Autodesk Inventor part; units mm, degrees
ref_plane "YZ Plane" through (0, 0, 0) normal (1, 0, 0) x (0, 1, 0)
ref_plane "XZ Plane" through (0, 0, 0) normal (0, 1, 0) x (-1, 0, 0)
ref_plane "XY Plane" through (0, 0, 0) normal (0, 0, 1) x (1, 0, 0)
sketch "Sketch1" plane through (0, 0, 0) normal (0, 1, 0) x (-1, 0, 0)
  line L0 (0.25, 0.25) -> (-0.25, 0.25)
  line L1 (-0.25, 0.25) -> (-0.25, -0.25)
  line L2 (-0.25, -0.25) -> (0.25, -0.25)
  line L3 (0.25, -0.25) -> (0.25, 0.25)
  line L4 (0.25, 0.25) -> (-0.25, -0.25) construction
  line L5 (-0.25, 0.25) -> (0.25, -0.25) construction
  point P0 (0, 0)
  dimension "d0" = 0.5
  dimension "d1" = 0.5
extrude "Extrusion1" add sketch "Sketch1" along normal blind 11.75
sketch "Sketch2" plane through (-0.25, 0, 0.25) normal (0, 0, 1) x (1, 0, 0)
  line L0 (0, 0) -> (0.5, 0)
  line L1 (0.5, 0) -> (0.5, 11.75)
  line L2 (0, 11.75) -> (0.5, 11.75)
  line L3 (0, 0) -> (0, 11.75)
  line L4 (0, 11.75) -> (0.5, 11.75)
  line L5 (0.5, 11.75) -> (0.5, 11.25)
  line L6 (0.5, 11.25) -> (0, 11.25)
  line L7 (0, 11.25) -> (0, 11.75)
  point P0 (0.25, 0)
  point P1 (0, 11.25)
  dimension "d10" = 0.5
extrude "Extrusion2" add sketch "Sketch2" along normal blind 3.3 contours L3 L2 L1 L6
properties part number "switch-wire"
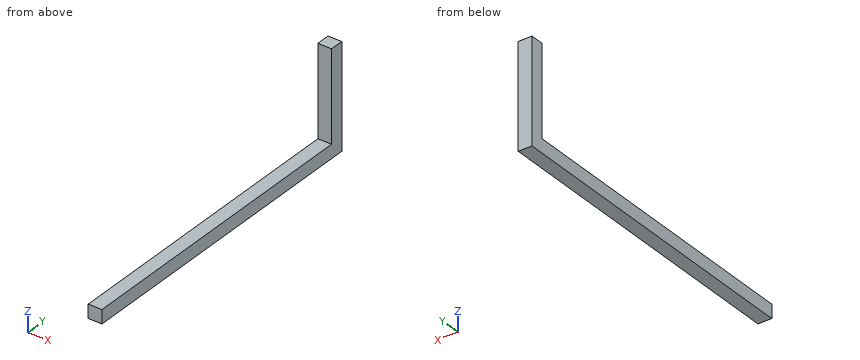
Geometry: final body of the model. Coordinates: model frame, mm. Round coordinates to 2 decimals unless told otherwise and drop trailing zeros. Write each loop counter-clockwise with the first axis right and the second up, starting at its lowest first coordinate (ties: lowest second). Pieces come first, ordered by that corner, then holes. Notation, with made-up numbers: (73, -29) -> (119, -29) arc R21 ccw to (119, -25) -> close; hole circle Ø11 at (41.5, -7). An arc over 180 degrees is marked (long way). Use CSV: the item, a comma, the result in double quotes. Start each with the question number.
Q1. Section C-C (z = 1.5). Return loops of the section in (x, y), plus the area to 3 significant figures.
Q2. Line query: L1, parallel to Z at x = -0.1, y = 9; L2, parallel to Y at x = 0.15, z = 1.85. Output: solid intervals per line, ascending.
Q3. Section A-A (y = 8.5). Return loops of the section in (x, z), plus the area to 3 significant figures.
Q4. Section B-B (x = -0.1). Return loops of the section in (y, z), plus the area to 4 significant figures.
Result sheet:
1,outline,"(-0.25, 11.25) -> (0.25, 11.25) -> (0.25, 11.75) -> (-0.25, 11.75) -> close"
1,area,"0.250 mm²"
2,L1,"-0.25 to 0.25"
2,L2,"11.25 to 11.75"
3,outline,"(-0.25, -0.25) -> (0.25, -0.25) -> (0.25, 0.25) -> (-0.25, 0.25) -> close"
3,area,"0.250 mm²"
4,outline,"(0, -0.25) -> (11.75, -0.25) -> (11.75, 3.55) -> (11.25, 3.55) -> (11.25, 0.25) -> (0, 0.25) -> close"
4,area,"7.525 mm²"
